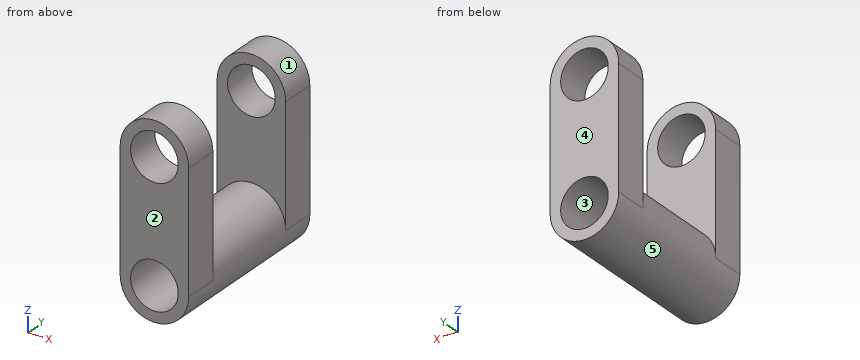
```python
from build123d import *

# Parameters (mm, degrees)
F0_R     = 17.243365
F1_DEPTH = 25.4
F2_DEPTH = 38.354


with BuildPart() as f1:
    # F0 (on Front) → F1 (new body)
    with BuildSketch(Plane.XZ):
        with BuildLine():
            ThreePointArc((29.55677, -59.970262), (4.711947, -35.125439), (-20.132875, -59.970262))
            ThreePointArc((-20.132875, -59.970262), (4.711947, -84.815084), (29.55677, -59.970262))
        make_face()
        with Locations((4.711947, -59.970262)):
            Circle(F0_R, mode=Mode.SUBTRACT)
        with BuildLine():
            ThreePointArc((29.55677, 26.986618), (4.711947, 2.141795), (-20.132875, 26.986618))
            Line((-20.132875, 26.986618), (-20.132875, -59.970262))
            ThreePointArc((-20.132875, -59.970262), (4.711947, -35.125439), (29.55677, -59.970262))
            Line((29.55677, -59.970262), (29.55677, 26.986618))
        make_face()
        with BuildLine():
            ThreePointArc((29.55677, 26.986618), (4.711947, 51.83144), (-20.132875, 26.986618))
            ThreePointArc((-20.132875, 26.986618), (4.711947, 2.141795), (29.55677, 26.986618))
        make_face()
        with Locations((4.711947, 26.986618)):
            Circle(F0_R, mode=Mode.SUBTRACT)
    extrude(amount=-F1_DEPTH)

    # F0 (on Front) → F2 (join)
    with BuildSketch(Plane.XZ):
        with BuildLine():
            ThreePointArc((29.55677, -59.970262), (4.711947, -35.125439), (-20.132875, -59.970262))
            ThreePointArc((-20.132875, -59.970262), (4.711947, -84.815084), (29.55677, -59.970262))
        make_face()
        with Locations((4.711947, -59.970262)):
            Circle(F0_R, mode=Mode.SUBTRACT)
    extrude(amount=F2_DEPTH)

    # F3: F1 across face


with BuildPart() as f1_1:
    add(f1.part)
    add(f1.part.mirror(Plane(origin=(4.711947, -38.354, -59.970262), x_dir=(1, 0, 0), z_dir=(0, -1, 0))))


solid = f1_1.part
```
Geometry check sheet. Reference: the model listing, model coordinates, mm. Face numbers are marked on the shaded views. A direction names the side the tool comes from. Coordinates: 2 decimals unless noted, no trailing zeros. Write each loop counter-clockwise with the first axis right and the second up, starting at its lowest first coordinate (ties: lowest second). Pieces come first, ordered by that corner, then holes. Notation, with made-up numbers: M 26,73 L 47,73 A14 ccw 47,77 Z; hole C 35.5,34.25 d8. An arc over 180 degrees is marked long. Use one line per item in the form item = value. Start each with the question number.
1) Section check A-A on z = -0.5. Enter the section's corners in (x, y).
2) Go/stop test with flat-tipped pins: pin 1 Ø1.5 at (x, y) = (24, 3.5) entering from -Z; pin 2 Ø1.5 at (x, y) = (8.5, -80.5) entering from -Z; pin 3 Ø6 at (x, y) = (-11, -33) entering from +Z. Record where each tip stops, or that it passes through.
3) Set-up check for the marked faces 4 and 5: record each of +Z, -Z, +X, -X, +Y, -Y from which the full face is reachable in a straight line by a thin tool's end or side.
4) Release check for a two-part mould opening along X. For the marked faces 1, 2 and 3 record: pulls with the +X half, pulls with the -X half, needs draft (parallel to the pull), parting line crosses it, or undercut.
5) Section check C-C on y = -83. Enter the section's corners in (x, z).
6) Section check B-B on x = -5.5. Enter the section's corners in (y, z).
7) Thickness scan on probe 1 along Y at (x, z) = (24, -5); probe 2 along Z at (x, y) = (16, 17.5); probe 3 along Z at (x, y) = (19, 19). Record the ranges inside material, lowest first. Write a range as from..to.
8) Section check D-D on z = -49. Enter the section's corners in (x, y), and give its area (3 significant figures).
Responses:
q1.outline = M -20.13,-102.11 L 29.56,-102.11 L 29.56,-76.71 L -20.13,-76.71 Z; M -20.13,0 L 29.56,0 L 29.56,25.4 L -20.13,25.4 Z
q2.pin_1 = -76.51
q2.pin_2 = -84.63
q2.pin_3 = -38.62
q3.face_4 = +Z, -Z, +X, -X, +Y
q3.face_5 = none
q4.face_1 = parting line crosses it
q4.face_2 = needs draft
q4.face_3 = undercut
q5.outline = M -20.13,-59.97 A24.84 ccw 29.56,-59.97 L 29.56,26.99 A24.84 ccw -20.13,26.99 Z; hole C 4.71,-59.97 d34.49; hole C 4.71,26.99 d34.49
q6.outline = M -102.11,-82.62 L 25.4,-82.62 L 25.4,-73.86 L -102.11,-73.86 Z; M -102.11,-46.08 L 25.4,-46.08 L 25.4,13.09 L 0,13.09 L 0,-37.32 L -76.71,-37.32 L -76.71,13.09 L -102.11,13.09 Z; M -102.11,40.88 L -76.71,40.88 L -76.71,49.64 L -102.11,49.64 Z; M 0,40.88 L 25.4,40.88 L 25.4,49.64 L 0,49.64 Z
q7.probe_1 = -102.11..-76.71, 0..25.4
q7.probe_2 = -82.1..-73.01, -46.94..13.95, 40.02..49.12
q7.probe_3 = -80.3..-69.62, -50.32..17.33, 36.64..47.31
q8.outline = M -20.13,-102.11 L -8.59,-102.11 L -8.59,25.4 L -20.13,25.4 L -20.13,0 L -17.58,0 L -17.58,-76.71 L -20.13,-76.71 Z; M 18.02,-102.11 L 29.56,-102.11 L 29.56,-76.71 L 27,-76.71 L 27,0 L 29.56,0 L 29.56,25.4 L 18.02,25.4 Z
q8.area = 2,550 mm2
